Part model, mm, in its own coordinate system. Face numbers are marked on the shaded views. A direction names the side the tool comes from. Round coordinates to 2 decimals unless told otherwise and drop trailing zeros. Write each loop counter-clockwise with the first axis right and the second up, starting at its lowest first coordinate (ties: lowest second). Pieces come first, ordered by that corner, then holes. Notation, with made-up numbers: (-33, 38.25) -> (17, 38.25) arc R10 ccw to (17, 44.25) -> close; hole circle Ø4 at (-15.5, -39.5). An arc over 180 degrees is marked (long way). Use CSV: the item, a comma, the result in double quotes. Start each with the question number.
(1) Saw through at A-A (z = 23). Give the cut face in (x, y), plus the area to 3 significant figures.
(2) Which spindle directions (+Z, -Z, +X, -X, +Y, -Y) get a long thin tool onto all of the face, cutting with end or side? Do the marked faces 4, 5, 6 and 7. Say none if no direction does.
(3) Two-plate mould, pull along Y, no slides. Class the marked faces 1, 2 and 3: released by +Y, released by -Y, zero draft, split by the parting line, or undercut.
(4) Drop flat-ended pins along their axis: pin 1 (1.8 mm diameter, centred on y = -3, z = 26, fed in from +X); pin 2 (3 mm diameter, centred on y = -1.5, z = 16, fed in from +X); pin 3 (1 mm diameter, centred on x = 3.5, y = -2, fed in from -Z). Give the stop position or say it passes through.
(5) Probe line 1 (X direction, y = 0, z = 14.75); line 2 (Y direction, x = 0, z = 15.75); line 3 (Y direction, x = 0, z = 9.25). List the from-to ranges inside material, lowest first. Write a range as [from, to].
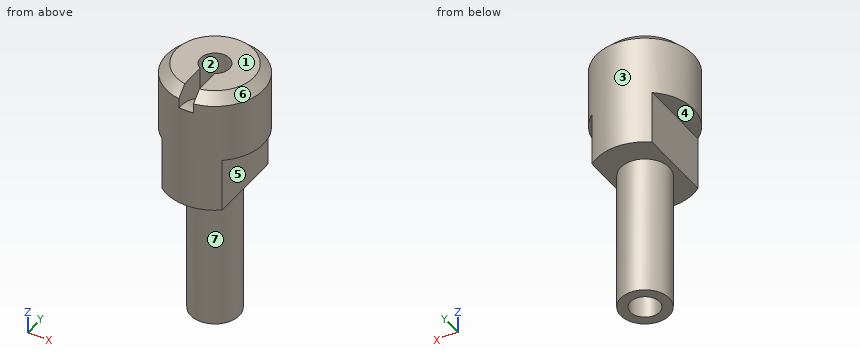
Autodesk Fusion 360 part; units mm, degrees
sketch "Sketch1" plane through (0, 0, 0) normal (0, 0, 1) x (1, 0, 0)
  circle A0 centre (0, 0) radius 2.5
  circle A1 centre (0, 0) radius 1.5
  dimension "d1" = 5
  dimension "d2" = 3
extrude "Extrude1" add sketch "Sketch1" along normal blind 20
sketch "Sketch2" plane through (0, 0, 20) normal (0, 0, 1) x (-1, 0, 0)
  circle A0 centre (0, 0) radius 1.5
  circle A1 centre (0, 0) radius 2.5
  circle A2 centre (0, 0) radius 5
  dimension "d5" = 2.5
extrude "Extrude2" add sketch "Sketch2" along normal blind 7 contours A1 | A2
sketch "Sketch3" plane through (0, 0, 0) normal (0, 1, 0) x (1, 0, 0)
  line L0 (-5, -27) -> (5, -27)
  line L1 (0, -27) -> (0, -20) construction
  line L2 (-5, -20) -> (5, -20)
  line L3 (-0.75, -27) -> (0.75, -27)
  line L4 (0.75, -27) -> (0.75, -25)
  line L5 (0.75, -25) -> (-0.75, -25)
  line L6 (-0.75, -25) -> (-0.75, -27)
  dimension "d8" = 1.5
  dimension "d9" = 2
extrude "Extrude3" cut sketch "Sketch3" against normal blind 6
sketch "Sketch4" plane through (0, 0, 0) normal (1, 0, 0) x (0, 1, 0)
  line L0 (-1.299, 27) -> (-4.9434, 27)
  line L1 (-1.299, 27) -> (1.5, 27)
  line L2 (-1.299, 25) -> (-4.9434, 25)
  line L3 (-1.299, 25) -> (-1.299, 23.4446)
  arc A0 (-1.299, 23.4446) -> (-4.9434, 25) centre (-4.9434, 19.9527) ccw
extrude "Extrude4" cut sketch "Sketch4" along normal blind 0.75 and the other way blind 0.75
chamfer "Chamfer1" distance 1 angle 45 1 edges at (0, 5, 27)
sketch "Sketch5" plane through (0, 0, 20) normal (0, 0, -1) x (1, 0, 0)
  circle A0 centre (0, 0) radius 5
  circle A1 centre (0, 0) radius 2.5
  circle A2 centre (0, 0) radius 5
  line L0 (-3.1, 3.923) -> (-3.1, -3.923)
  line L1 (3.1, 3.923) -> (3.1, -3.923)
  line L2 (0, -5) -> (0, 5) construction
  dimension "d19" = 6.2
extrude "Extrude5" add sketch "Sketch5" along normal blind 5.5 contours A0 A2 L0 L1
Answers:
1,outline,"circle Ø10 at (0, 0); hole circle Ø3 at (0, 0)"
1,area,"71.5 mm²"
2,face 4,"-Z, -X, +Y, -Y"
2,face 5,"-Z, +X, +Y, -Y"
2,face 6,"+Z"
2,face 7,"-Z"
3,face 1,"zero draft"
3,face 2,"undercut"
3,face 3,"split by the parting line"
4,pin 1,"stops at x = 4.54"
4,pin 2,"stops at x = 3.1"
4,pin 3,"stops at z = 14.5"
5,line 1,"x = [-3.1, -1.5], [1.5, 3.1]"
5,line 2,"y = [-5, -1.5], [1.5, 5]"
5,line 3,"y = [-2.5, -1.5], [1.5, 2.5]"
